Source: CAD feature listing. Evaluate the final solid. Frame: model axes, mm. Face numbers are marked on the shaded views. A direction names the side the tool comes from. Coordinates: 2 decimals unless noted, no trailing zeros. Write each loop counter-clockwise with the first axis right and the second up, starting at its lowest first coordinate (ties: lowest second). Pieces come first, ordered by that corner, then holes. Notation, with made-up numbers: (38, -0.5) - (52, -0.5) arc R22 cw to (52, 6.5) - close; hole circle Ø6 at (-35, 28). An arc over 180 degrees is marked (long way). One line per item, written item: value.
from build123d import *

# Parameters (mm, degrees)
F1_DEPTH  = 67.15461
F2_DEPTH  = 69.79008
F3_R      = 51.747749
F3_R_2    = 43.976375
F4_DEPTH  = 17.61725
F5_W      = 52.022107
F5_H      = 22.369506
F5_H_2    = 19.664356
F5_H_3    = 6.866917
F6_DEPTH  = 25.7345
F7_W      = 52.022105
F7_H      = 4.994122
F8_DEPTH  = 25.82881
F9_R      = 52.073065
F10_DEPTH = 34.79581


with BuildPart() as f1:
    # F0 (on Front) → F1 (new body)
    with BuildSketch(Plane.XZ):
        with BuildLine():
            ThreePointArc((15.025515, 49.610047), (1.396386, 43.41215), (-11.806262, 50.473112))
            ThreePointArc((-11.806262, 50.473112), (-14.424876, 49.788009), (-17.004157, 48.967147))
            ThreePointArc((-17.004157, 48.967147), (-24.387322, 35.941942), (-39.218818, 33.894058))
            ThreePointArc((-39.218818, 33.894058), (-40.934627, 31.800616), (-42.538819, 29.620462))
            ThreePointArc((-42.538819, 29.620462), (-40.855901, 14.743134), (-51.651118, 4.368627))
            ThreePointArc((-51.651118, 4.368627), (-51.808742, 1.666469), (-51.825098, -1.040233))
            ThreePointArc((-51.825098, -1.040233), (-41.718915, -12.08705), (-44.354446, -26.825472))
            ThreePointArc((-44.354446, -26.825472), (-42.893678, -29.104213), (-41.315951, -31.303595))
            ThreePointArc((-41.315951, -31.303595), (-26.646721, -34.300392), (-20.115884, -47.773152))
            ThreePointArc((-20.115884, -47.773152), (-17.594688, -48.758074), (-15.025515, -49.610047))
            ThreePointArc((-15.025515, -49.610047), (-1.396386, -43.41215), (11.806262, -50.473112))
            ThreePointArc((11.806262, -50.473112), (14.424876, -49.788009), (17.004157, -48.967147))
            ThreePointArc((17.004157, -48.967147), (24.387322, -35.941942), (39.218818, -33.894058))
            ThreePointArc((39.218818, -33.894058), (40.934627, -31.800616), (42.538819, -29.620462))
            ThreePointArc((42.538819, -29.620462), (40.855901, -14.743134), (51.651118, -4.368627))
            ThreePointArc((51.651118, -4.368627), (51.808742, -1.666469), (51.825098, 1.040233))
            ThreePointArc((51.825098, 1.040233), (41.718915, 12.08705), (44.354446, 26.825472))
            ThreePointArc((44.354446, 26.825472), (42.893678, 29.104213), (41.315951, 31.303595))
            ThreePointArc((41.315951, 31.303595), (26.646721, 34.300392), (20.115884, 47.773152))
            ThreePointArc((20.115884, 47.773152), (17.594688, 48.758074), (15.025515, 49.610047))
        make_face()
    extrude(amount=F1_DEPTH)

    # F1_face (on face) → F2 (join)
    with BuildSketch(Plane.XZ.offset(67.15461)):
        with BuildLine():
            ThreePointArc((41.315951, 31.303595), (26.646721, 34.300392), (20.115884, 47.773152))
            ThreePointArc((20.115884, 47.773152), (17.594688, 48.758074), (15.025515, 49.610047))
            ThreePointArc((15.025515, 49.610047), (1.396386, 43.41215), (-11.806262, 50.473112))
            ThreePointArc((-11.806262, 50.473112), (-14.424876, 49.788009), (-17.004157, 48.967147))
            ThreePointArc((-17.004157, 48.967147), (-24.387322, 35.941942), (-39.218818, 33.894058))
            ThreePointArc((-39.218818, 33.894058), (-40.934627, 31.800616), (-42.538819, 29.620462))
            ThreePointArc((-42.538819, 29.620462), (-40.855901, 14.743134), (-51.651118, 4.368627))
            ThreePointArc((-51.651118, 4.368627), (-51.808742, 1.666469), (-51.825098, -1.040233))
            ThreePointArc((-51.825098, -1.040233), (-41.718915, -12.08705), (-44.354446, -26.825472))
            ThreePointArc((-44.354446, -26.825472), (-42.893678, -29.104213), (-41.315951, -31.303595))
            ThreePointArc((-41.315951, -31.303595), (-26.646721, -34.300392), (-20.115884, -47.773152))
            ThreePointArc((-20.115884, -47.773152), (-17.594688, -48.758074), (-15.025515, -49.610047))
            ThreePointArc((-15.025515, -49.610047), (-1.396386, -43.41215), (11.806262, -50.473112))
            ThreePointArc((11.806262, -50.473112), (14.424876, -49.788009), (17.004157, -48.967147))
            ThreePointArc((17.004157, -48.967147), (24.387322, -35.941942), (39.218818, -33.894058))
            ThreePointArc((39.218818, -33.894058), (40.934627, -31.800616), (42.538819, -29.620462))
            ThreePointArc((42.538819, -29.620462), (40.855901, -14.743134), (51.651118, -4.368627))
            ThreePointArc((51.651118, -4.368627), (51.808742, -1.666469), (51.825098, 1.040233))
            ThreePointArc((51.825098, 1.040233), (41.718915, 12.08705), (44.354446, 26.825472))
            ThreePointArc((44.354446, 26.825472), (42.893678, 29.104213), (41.315951, 31.303595))
        make_face()
        with BuildLine():
            ThreePointArc((20.115884, 47.773152), (26.646721, 34.300392), (41.315951, 31.303595))
            ThreePointArc((41.315951, 31.303595), (42.893678, 29.104213), (44.354446, 26.825472))
            ThreePointArc((44.354446, 26.825472), (41.718915, 12.08705), (51.825098, 1.040233))
            ThreePointArc((51.825098, 1.040233), (51.808742, -1.666469), (51.651118, -4.368627))
            ThreePointArc((51.651118, -4.368627), (40.855901, -14.743134), (42.538819, -29.620462))
            ThreePointArc((42.538819, -29.620462), (40.934627, -31.800616), (39.218818, -33.894058))
            ThreePointArc((39.218818, -33.894058), (24.387322, -35.941942), (17.004157, -48.967147))
            ThreePointArc((17.004157, -48.967147), (14.424876, -49.788009), (11.806262, -50.473112))
            ThreePointArc((11.806262, -50.473112), (-1.396386, -43.41215), (-15.025515, -49.610047))
            ThreePointArc((-15.025515, -49.610047), (-17.594688, -48.758074), (-20.115884, -47.773152))
            ThreePointArc((-20.115884, -47.773152), (-26.646721, -34.300392), (-41.315951, -31.303595))
            ThreePointArc((-41.315951, -31.303595), (-42.893678, -29.104213), (-44.354446, -26.825472))
            ThreePointArc((-44.354446, -26.825472), (-41.718915, -12.08705), (-51.825098, -1.040233))
            ThreePointArc((-51.825098, -1.040233), (-51.808742, 1.666469), (-51.651118, 4.368627))
            ThreePointArc((-51.651118, 4.368627), (-40.855901, 14.743134), (-42.538819, 29.620462))
            ThreePointArc((-42.538819, 29.620462), (-40.934627, 31.800616), (-39.218818, 33.894058))
            ThreePointArc((-39.218818, 33.894058), (-24.387322, 35.941942), (-17.004157, 48.967147))
            ThreePointArc((-17.004157, 48.967147), (-14.424876, 49.788009), (-11.806262, 50.473112))
            ThreePointArc((-11.806262, 50.473112), (1.396386, 43.41215), (15.025515, 49.610047))
            ThreePointArc((15.025515, 49.610047), (17.594688, 48.758074), (20.115884, 47.773152))
        make_face()
    extrude(amount=F2_DEPTH)

    # F3 (on Front) → F4 (join)
    with BuildSketch(Plane.XZ):
        Circle(F3_R)
        Circle(F3_R_2, mode=Mode.SUBTRACT)
    extrude(amount=-F4_DEPTH)

    # F5 (on Front) → F6 (join)
    with BuildSketch(Plane.XZ):
        with Locations((-0.104043, -11.184753)):
            Rectangle(F5_W, F5_H)
        with Locations((-0.104043, 9.832178)):
            Rectangle(F5_W, F5_H_2)
        with Locations((-0.104043, 23.097814)):
            Rectangle(F5_W, F5_H_3)
    extrude(amount=-F6_DEPTH)

    # F7 (on Front) → F8 (join)
    with BuildSketch(Plane.XZ):
        with Locations((-0.312131, -24.866567)):
            Rectangle(F7_W, F7_H)
    extrude(amount=-F8_DEPTH)

    # F9 (on face) → F10 (join)
    with BuildSketch(Plane.XZ.offset(136.94469)):
        Circle(F9_R)
    extrude(amount=-F10_DEPTH)


solid = f1.part
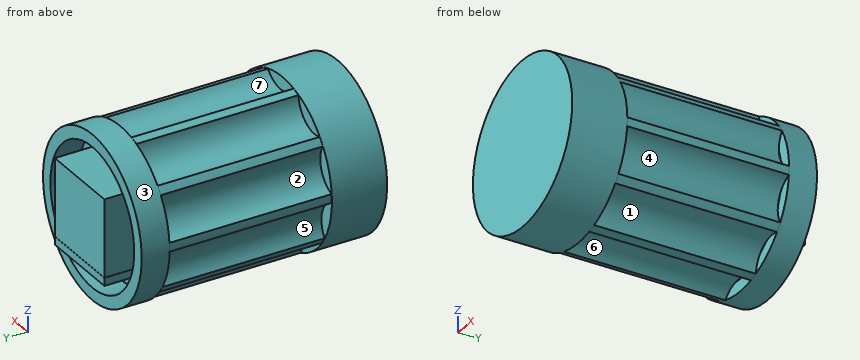
1) Material intervals for line 1 (Z direction, x = 0, y = 6); line 2 (X direction, y = 8.75, z = 0); line 3 (Y direction, x = 2, z = 38), sorted ascending.
Values found:
line 1: -51.75 to -43.98, -27.36 to 26.53, 43.98 to 51.75
line 2: -51.75 to -43.98, -26.12 to 25.91, 43.98 to 51.75
line 3: -136.94 to 0
2) Reachability of the marked faces 1, 2, 3 and 4 from +Z, -Z, +X, -X, +Y, -Y: full face, straight path, thin tool, end or side. Return the list, or none.
Values found:
face 1: -Z
face 2: -X
face 3: +Y
face 4: +X
3) Section query A-A on y = 15. Output: boundary loops of the cut face in (x, z), then the cut area to 3 significant figures.
Values found:
outline: circle Ø103.5 at (0, 0); (-26.32, -27.36) - (25.7, -27.36) - (25.7, -22.37) - (25.91, -22.37) - (25.91, 26.53) - (-26.12, 26.53) - (-26.12, -22.37) - (-26.32, -22.37) - close; hole circle Ø87.95 at (0, 0)
area: 5,140 mm2
4) Draft query along Z for the marked faces 5, 6 and 7. Return one class per face: released by +Z, released by -Z, zero draft, split by the parting line, or undercut.
Values found:
face 5: undercut
face 6: released by -Z
face 7: released by +Z
5) Section query C-C on z = 20.5. Output: boundary loops of the cut face in (x, y), then the cut area to 3 significant figures.
Values found:
outline: (-47.87, -136.94) - (47.87, -136.94) - (47.87, -102.15) - (41.46, -102.15) - (41.46, 0) - (47.51, 0) - (47.51, 17.62) - (38.91, 17.62) - (38.91, 0) - (25.91, 0) - (25.91, 25.73) - (-26.12, 25.73) - (-26.12, 0) - (-38.91, 0) - (-38.91, 17.62) - (-47.51, 17.62) - (-47.51, 0) - (-39.85, 0) - (-39.85, -102.15) - (-47.87, -102.15) - close
area: 13,300 mm2
6) Contact query for flat-ended pins moving along their axis: P1, Ø2, axis at x = 11.5, y = -96, coming from the +Z side; P2, Ø12, axis at x = 28, y = -53.5, coming from the +Z side; P3, Ø8, axis at x = 7, y = -64.5, coming from the +Z side; P4, Ø5, axis at x = 35, z = 43, coming from the -Y side. Output: stop coordinate, or through.
Values found:
P1: z = 47.11
P2: z = 39.89
P3: z = 46.04
P4: through
7) Section query B-B on y = -54.5. Output: boundary loops of the cut face in (x, z).
Values found:
outline: (-51.83, -1.04) arc R16.9 cw to (-44.35, -26.83) arc R51.84 ccw to (-41.32, -31.3) arc R16.9 cw to (-20.12, -47.77) arc R51.84 ccw to (-15.03, -49.61) arc R16.9 cw to (11.81, -50.47) arc R51.84 ccw to (17, -48.97) arc R16.9 cw to (39.22, -33.89) arc R51.84 ccw to (42.54, -29.62) arc R16.9 cw to (51.65, -4.37) arc R51.84 ccw to (51.83, 1.04) arc R16.9 cw to (44.35, 26.83) arc R51.84 ccw to (41.32, 31.3) arc R16.9 cw to (20.12, 47.77) arc R51.84 ccw to (15.03, 49.61) arc R16.9 cw to (-11.81, 50.47) arc R51.84 ccw to (-17, 48.97) arc R16.9 cw to (-39.22, 33.89) arc R51.84 ccw to (-42.54, 29.62) arc R16.9 cw to (-51.65, 4.37) arc R51.84 ccw to start
8) Section query D-D on x = 0. Output: boundary loops of the cut face in (y, z).
Values found:
outline: (-136.94, -52.07) - (-102.15, -52.07) - (-102.15, -43.52) - (0, -43.52) - (0, -27.36) - (25.83, -27.36) - (25.83, -22.37) - (25.73, -22.37) - (25.73, 26.53) - (0, 26.53) - (0, 43.52) - (-102.15, 43.52) - (-102.15, 52.07) - (-136.94, 52.07) - close; (0, -51.75) - (17.62, -51.75) - (17.62, -43.98) - (0, -43.98) - close; (0, 43.98) - (17.62, 43.98) - (17.62, 51.75) - (0, 51.75) - close
